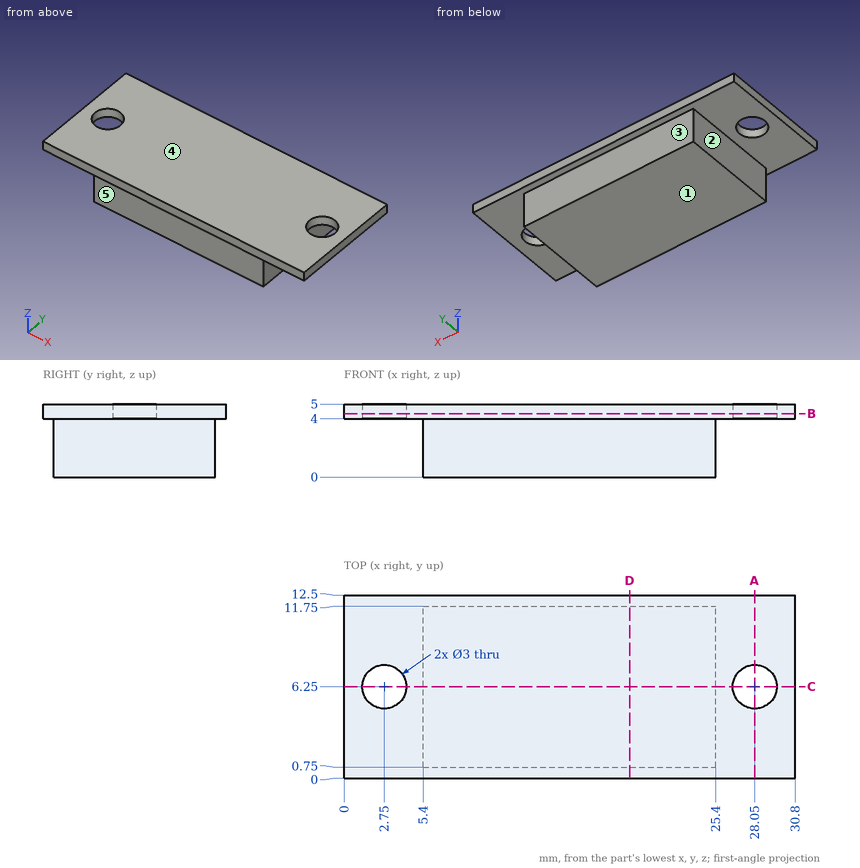
Here's the drawing with two shaded views (mm, measured from the low corner). I have some questions. A direction names the side the tool comes from. Coordinates: 2 decimals unless noted, no trailing zeros. Write each loop counter-clockwise with the first axis right and the second up, starting at its lowest first coordinate (ties: lowest second). Pieces come first, ordered by that corner, then holes. Notation, with made-up numbers: (-21.5, 88) -> (-0.5, 88) arc R17 ccw to (-0.5, 117) -> close; hole circle Ø4 at (26, 12.5). An arc over 180 degrees is marked (long way). Use a Markdown table: item, result. Add a question column.
(1) If we section it at A-A, the plane x = 28.05: Write out the boundary of the cut face in (y, z), and give its area (3 significant figures).
(2) If we section it at C-C, the plane y = 6.25: Write out the boundary of the cut face in (x, z), and give its area (3 significant figures).
(3) If we section it at D-D, the plane x = 19.5: Write out the boundary of the cut face in (y, z).
(4) I'm going to push flat-ended pins straight in: P1, Ø3, axis at y = 5, z = 2, coming from the +X side; P2, Ø2.5, axis at x = 28.05, y = 6.25, coming from the +Z side; P3, Ø2, axis at y = 6, z = 2.5, coming from the -X side; P4, Ø2, axis at x = 4.5, z = 2.5, coming from the +Y side. Where does each tip first touch, or does it pass through?
(5) Please list where these lines run through material, in increasing order: line 1 (Y direction, x = 28.05, z = 4.3); line 2 (Z direction, x = 5, y = 6); line 3 (X direction, y = 2.25, z = 2.55).
(6) For the marked faces 1, 2, 3, 4 and 5, which set-ups out of +Z, -Z, +X, -X, +Y, -Y let a thin tool reach every point of the face, with its end or its side?
(7) If we section it at B-B, the plane z = 4.35: Write out the boundary of the cut face in (x, y), and give its area (3 significant figures).
Outcome:
| question | item | result |
|---|---|---|
| 1 | outline | (0, 4) -> (4.75, 4) -> (4.75, 5) -> (0, 5) -> close; (7.75, 4) -> (12.5, 4) -> (12.5, 5) -> (7.75, 5) -> close |
| 1 | area | 9.50 mm^2 |
| 2 | outline | (0, 4) -> (1.25, 4) -> (1.25, 5) -> (0, 5) -> close; (4.25, 4) -> (5.4, 4) -> (5.4, 0) -> (25.4, 0) -> (25.4, 4) -> (26.55, 4) -> (26.55, 5) -> (4.25, 5) -> close; (29.55, 4) -> (30.8, 4) -> (30.8, 5) -> (29.55, 5) -> close |
| 2 | area | 105 mm^2 |
| 3 | outline | (0, 4) -> (0.75, 4) -> (0.75, 0) -> (11.75, 0) -> (11.75, 4) -> (12.5, 4) -> (12.5, 5) -> (0, 5) -> close |
| 4 | P1 | stops at x = 25.4 |
| 4 | P2 | passes through |
| 4 | P3 | stops at x = 5.4 |
| 4 | P4 | stops at y = 11.75 |
| 5 | line 1 | y = 0 to 4.75, 7.75 to 12.5 |
| 5 | line 2 | z = 4 to 5 |
| 5 | line 3 | x = 5.4 to 25.4 |
| 6 | face 1 | -Z, +X, -X, +Y, -Y |
| 6 | face 2 | -Z, -X, +Y, -Y |
| 6 | face 3 | -Z, +X, -X, +Y |
| 6 | face 4 | +Z, +X, -X, +Y, -Y |
| 6 | face 5 | -Z, +X, -X, -Y |
| 7 | outline | (0, 0) -> (30.8, 0) -> (30.8, 12.5) -> (0, 12.5) -> close; hole circle Ø3 at (2.75, 6.25); hole circle Ø3 at (28.05, 6.25) |
| 7 | area | 371 mm^2 |
